Work out the finished part from the listing and answer in its coordinate system (mm). A direction names the side the tool comes from. Coordinates: 2 decimals unless noted, no trailing zeros. Order: outer loops, then holes, each group sorted by start corner. A loop starts at its lowest first (then second) coordinate and runs counter-clockwise, first axis right, second up. Notation, with made-up numbers: M 48,36.5 L 74,36.5 A20 ccw 74,49.5 Z; hole C 48.5,84 d8. An arc over 180 degrees is marked long. Write item = value, one per line. Start each with the question number.
Q1. Determine the mould class of faces 1 (the flat face through (9, 100, -89.732)), 2 (the flat face through (7, 5, 24)), 3 (the flat face through (117.297, 99, 27)) for opening direction Z: released by +Z, released by -Z, zero draft, split by the parting line, or undercut.
Q2. Find section D-D on x = 54.5. Give the vertices of the cut face in (y, z).
Q3. Find section B-B on y = 27. Give the vertices of the cut face in (x, z), and give its area (3 significant figures).
Q4. This flat-tipped pin is pushed along its axis until it touches: P1, Ø12, axis at x = -44, z = 99.5, coming from the +Y side. Where does it stop, or does it pass through?
Q5. Find section C-C on z = -8.5. Give the vertices of the cut face in (x, y).
Q6. Straight lines are drawn through the part: line 1 along Z through (x, y) = (114, 35); line 2 along Z through (x, y) = (-17.5, 157.5); line 3 along X through (y, z) = (25, 75). For each, find the intervals that lie inside material, in ascending order.
Q7. A tool of negligible diameter and unlimited length cuts with its end or side. For faces 4 (the flat face through (9, 100, 140.268)), 5 (the flat face through (7, 104, -84.732)), from which of +Z, -Z, +X, -X, +Y, -Y can it reach the whole face along a straight path? Write none if from no direction.
Q8. Find section A-A on y = 127.5. Give the vertices of the cut face in (x, z).
```python
from build123d import *

# Parameters (mm, degrees)
SKETCH1_W           = 217
SKETCH1_H           = 230
BOSS_EXTRUDE1_DEPTH = 200
SKETCH2_W           = 207
SKETCH2_H           = 220
CUT_EXTRUDE1_DEPTH  = 195
FILLET1_R           = 3
CUT_EXTRUDE2_DEPTH  = 5
CUT_EXTRUDE3_DEPTH  = 10


with BuildPart() as part:
    # Sketch1 → Boss-Extrude1 (new body)
    with BuildSketch(Plane(origin=(0, 0, 0), x_dir=(1, 0, 0), z_dir=(0, 1, 0))):
        with Locations((8.797297297, -25.267567568)):
            Rectangle(SKETCH1_W, SKETCH1_H)
    extrude(amount=BOSS_EXTRUDE1_DEPTH)

    # Sketch2 → Cut-Extrude1 (cut)
    with BuildSketch(Plane(origin=(0, 200, 0), x_dir=(1, 0, 0), z_dir=(0, 1, 0))):
        with Locations((8.797297297, -25.267567568)):
            Rectangle(SKETCH2_W, SKETCH2_H)
    extrude(amount=-CUT_EXTRUDE1_DEPTH, mode=Mode.SUBTRACT)

    # Fillet1
    fillet1_edges = [part.edges().sort_by_distance(p)[0] for p in [
        (8.797297297, 0, -89.732432432),
        (8.797297297, 0, 140.267567568),
        (-99.702702703, 0, 25.267567568),
        (-99.702702703, 100, -89.732432432),
        (-99.702702703, 100, 140.267567568),
    ]]
    fillet(fillet1_edges, radius=FILLET1_R)

    # Sketch3 → Cut-Extrude2 (cut)
    with BuildSketch(Plane(origin=(117.297297297, 0, 0), x_dir=(0, 0, -1), z_dir=(1, 0, 0))):
        with BuildLine():
            ThreePointArc((-105.267567568, 162.5), (-103.499800615, 163.232233047), (-102.767567568, 165))
            Line((-102.767567568, 165), (-105.267567568, 165))
            Line((-105.267567568, 165), (-105.267567568, 162.5))
        make_face()
        with BuildLine():
            Line((-105.267567568, 165), (-102.767567568, 165))
            ThreePointArc((-102.767567568, 165), (-107.035334521, 166.767766953), (-105.267567568, 162.5))
            Line((-105.267567568, 162.5), (-105.267567568, 165))
        make_face()
        with BuildLine():
            ThreePointArc((-105.267567568, 37.5), (-107.035334521, 33.232233047), (-102.767567568, 35))
            Line((-102.767567568, 35), (-105.267567568, 35))
            Line((-105.267567568, 35), (-105.267567568, 37.5))
        make_face()
        with BuildLine():
            Line((-105.267567568, 35), (-102.767567568, 35))
            ThreePointArc((-102.767567568, 35), (-103.499800615, 36.767766953), (-105.267567568, 37.5))
            Line((-105.267567568, 37.5), (-105.267567568, 35))
        make_face()
        with BuildLine():
            ThreePointArc((37.232432432, 35), (36.500199385, 36.767766953), (34.732432432, 37.5))
            Line((34.732432432, 37.5), (34.732432432, 35))
            Line((34.732432432, 35), (32.232432432, 35))
            ThreePointArc((32.232432432, 35), (34.732432432, 32.5), (37.232432432, 35))
        make_face()
        with BuildLine():
            Line((34.732432432, 35), (34.732432432, 37.5))
            ThreePointArc((34.732432432, 37.5), (32.964665479, 36.767766953), (32.232432432, 35))
            Line((32.232432432, 35), (34.732432432, 35))
        make_face()
        with BuildLine():
            Line((32.56180467, 102.425143832), (34.732432432, 101.184831324))
            Line((34.732432432, 101.184831324), (34.732432432, 98.684831324))
            ThreePointArc((34.732432432, 98.684831324), (36.500199385, 99.417064371), (37.232432432, 101.184831324))
            ThreePointArc((37.232432432, 101.184831324), (35.37408288, 103.601085595), (32.56180467, 102.425143832))
        make_face()
        with BuildLine():
            Line((34.732432432, 98.684831324), (34.732432432, 101.184831324))
            Line((34.732432432, 101.184831324), (32.56180467, 102.425143832))
            ThreePointArc((32.56180467, 102.425143832), (32.570167269, 99.929996927), (34.732432432, 98.684831324))
        make_face()
    extrude(amount=-CUT_EXTRUDE2_DEPTH, mode=Mode.SUBTRACT)

    # Sketch4 → Cut-Extrude3 (cut)
    with BuildSketch(Plane(origin=(117.297297297, 0, 0), x_dir=(0, 0, -1), z_dir=(1, 0, 0))):
        with BuildLine():
            Line((64.732432432, 102.133518404), (74.732432432, 102.133518404))
            ThreePointArc((74.732432432, 102.133518404), (78.267966338, 100.66905231), (79.732432432, 97.133518404))
            Line((79.732432432, 97.133518404), (79.732432432, 14.966834817))
            ThreePointArc((79.732432432, 14.966834817), (78.267966338, 11.431300911), (74.732432432, 9.966834817))
            Line((74.732432432, 9.966834817), (64.732432432, 9.966834817))
            ThreePointArc((64.732432432, 9.966834817), (61.196898526, 11.431300911), (59.732432432, 14.966834817))
            Line((59.732432432, 14.966834817), (59.732432432, 97.133518404))
            ThreePointArc((59.732432432, 97.133518404), (61.196898526, 100.66905231), (64.732432432, 102.133518404))
        make_face()
    extrude(amount=-CUT_EXTRUDE3_DEPTH, mode=Mode.SUBTRACT)


solid = part.part
```
Findings below:
q1.face_1 = released by -Z
q1.face_2 = undercut
q1.face_3 = zero draft
q2.outline = M 0,-86.73 A3 ccw 3,-89.73 L 200,-89.73 L 200,-84.73 L 5,-84.73 L 5,135.27 L 200,135.27 L 200,140.27 L 3,140.27 A3 ccw 0,137.27 Z
q3.outline = M -99.7,-86.73 A3 ccw -96.7,-89.73 L 117.3,-89.73 L 117.3,-79.73 L 112.3,-79.73 L 112.3,-84.73 L -94.7,-84.73 L -94.7,135.27 L 112.3,135.27 L 112.3,-59.73 L 117.3,-59.73 L 117.3,140.27 L -96.7,140.27 A3 ccw -99.7,137.27 Z
q3.area = 4,270 mm^2
q4.P1 = 5
q5.outline = M -99.7,3 A3 ccw -96.7,0 L 117.3,0 L 117.3,200 L 112.3,200 L 112.3,5 L -94.7,5 L -94.7,200 L -99.7,200 Z
q6.line_1 = -89.73 to -79.73, -59.73 to -37.23, -32.23 to 102.77, 107.77 to 140.27
q6.line_2 = -89.73 to -84.73, 135.27 to 140.27
q6.line_3 = -99.7 to -94.7, 112.3 to 117.3
q7.face_4 = +Z, +X, -X, +Y, -Y
q7.face_5 = +Y
q8.outline = M -99.7,-86.73 A3 ccw -96.7,-89.73 L 117.3,-89.73 L 117.3,140.27 L -96.7,140.27 A3 ccw -99.7,137.27 Z; hole M -94.7,-84.73 L 112.3,-84.73 L 112.3,135.27 L -94.7,135.27 Z
